```python
from build123d import *

# Parameters (mm, degrees)
SKETCH_1_W          = 220
SKETCH_1_H          = 45
EXTRUDE_1_DEPTH     = 6
EXTRUDE_2_DEPTH     = 35
SKETCH_5_W          = 4
SKETCH_5_H          = 3
CUT_EXTRUDE_3_DEPTH = 194.244663574
SKETCH_6_W          = 220
SKETCH_6_H          = 45
EXTRUDE_3_DEPTH     = 5
EXTRUDE_4_DEPTH     = 11
SKETCH_10_R         = 4.5
CUT_EXTRUDE_4_DEPTH = 172.992005628
FILLET_1_R          = 10
SKETCH_11_W         = 10
SKETCH_11_H         = 8
CUT_EXTRUDE_6_DEPTH = 35
SKETCH_18_W         = 228
SKETCH_18_H         = 45
EXTRUDE_5_DEPTH     = 1


with BuildPart() as part:
    # 草图1 → 凸台-拉伸1 (new body)
    with BuildSketch(Plane.XY):
        Rectangle(SKETCH_1_W, SKETCH_1_H)
    extrude(amount=EXTRUDE_1_DEPTH)

    # 草图2 → 凸台-拉伸2 (add)
    with BuildSketch(Plane.XY.offset(6)):
        Polygon((-77.5, 22.5), (77.5, 22.5), (77.5, 14.5), (75, 14.5), (-75, 14.5), (-77.5, 14.5), align=None)
        Polygon((-75, -14.5), (75, -14.5), (77.5, -14.5), (77.5, -22.5), (-77.5, -22.5), (-77.5, -14.5), align=None)
    extrude(amount=EXTRUDE_2_DEPTH)

    # 草图5 → 切除-拉伸3 (cut, through all)
    with BuildSketch(Plane.ZY.offset(77.5)):
        with Locations((11.5, -16)):
            Rectangle(SKETCH_5_W, SKETCH_5_H)
        with Locations((11.5, 16)):
            Rectangle(SKETCH_5_W, SKETCH_5_H)
    extrude(amount=-CUT_EXTRUDE_3_DEPTH, mode=Mode.SUBTRACT)

    # 草图6 → 凸台-拉伸3 (add)
    with BuildSketch(Plane(origin=(0, 0, 0), x_dir=(-1, 0, 0), z_dir=(0, 0, -1))):
        Rectangle(SKETCH_6_W, SKETCH_6_H)
    extrude(amount=EXTRUDE_3_DEPTH)

    # 草图9 → 凸台-拉伸4 (add)
    with BuildSketch(Plane(origin=(0, 0, -5), x_dir=(-1, 0, 0), z_dir=(0, 0, -1))):
        with BuildLine():
            Line((-110, -22.5), (-110, 22.5))
            Line((-110, 22.5), (-130, 22.5))
            Line((-130, 22.5), (-158.235294118, -30.441176471))
            ThreePointArc((-158.235294118, -30.441176471), (-152.058823529, -50.735294118), (-131.764705882, -44.558823529))
            Line((-131.764705882, -44.558823529), (-120, -22.5))
            Line((-120, -22.5), (-110, -22.5))
        make_face()
    extrude_4 = extrude(amount=-EXTRUDE_4_DEPTH)

    # 草图10 → 切除-拉伸4 (cut, through all)
    with BuildSketch(Plane.XY.offset(6)):
        with Locations((145, -37.5)):
            Circle(SKETCH_10_R)
    cut_extrude_4 = extrude(amount=-CUT_EXTRUDE_4_DEPTH, mode=Mode.SUBTRACT)

    # 镜向1: 凸台-拉伸4, 切除-拉伸4 across plane
    add(extrude_4.mirror(Plane(origin=(0, 0, 0), x_dir=(0, 0, 1), z_dir=(1, 0, 0))))
    add(cut_extrude_4.mirror(Plane(origin=(0, 0, 0), x_dir=(0, 0, 1), z_dir=(1, 0, 0))), mode=Mode.SUBTRACT)

    # 圆角1
    fillet_1_edges = [part.edges().sort_by_distance(p)[0] for p in [
        (-130, 22.5, 0.5),
        (-120, -22.5, 0.5),
        (130, 22.5, 0.5),
        (120, -22.5, 0.5),
    ]]
    fillet(fillet_1_edges, radius=FILLET_1_R)

    # 草图11 → 切除-拉伸6 (cut)
    with BuildSketch(Plane.XY.offset(41)):
        with Locations((-72.5, 18.5)):
            Rectangle(SKETCH_11_W, SKETCH_11_H)
        with Locations((72.5, 18.5)):
            Rectangle(SKETCH_11_W, SKETCH_11_H)
        with Locations((72.5, -18.5)):
            Rectangle(SKETCH_11_W, SKETCH_11_H)
        with Locations((-72.5, -18.5)):
            Rectangle(SKETCH_11_W, SKETCH_11_H)
    extrude(amount=-CUT_EXTRUDE_6_DEPTH, mode=Mode.SUBTRACT)

    # 草图18 → 凸台-拉伸5 (add)
    with BuildSketch(Plane(origin=(0, 0, -5), x_dir=(-1, 0, 0), z_dir=(0, 0, -1))):
        Rectangle(SKETCH_18_W, SKETCH_18_H)
    extrude(amount=EXTRUDE_5_DEPTH)


solid = part.part
```
Model file for the job. Use its own axes, mm. A direction names the side the tool comes from. Round coordinates to 2 decimals unless told otherwise and drop trailing zeros. Write each loop counter-clockwise with the first axis right and the second up, starting at its lowest first coordinate (ties: lowest second). Pieces come first, ordered by that corner, then holes. Notation, with made-up numbers: M 57,74 L 110,74 A13 cw 110,94 Z; hole C 56.25,69.25 d6. An arc over 180 degrees is marked long. Put each result on its own line as item: value.
Item 1: Tool access for faces 4 (the cylindrical face through (-119.21, -23.964, 0.577)), 5 (the flat face through (1, -14.5, 27)), 6 (the flat face through (67.5, -19, 24)): list every direction of +Z, -Z, +X, -X, +Y, -Y with a clear straight run to the whole face (end or side of a thin tool).
Responses:
face 4: +Z, -Z, -Y
face 5: +Z, +X, -X
face 6: +Z, +X, +Y, -Y
Item 2: Cut at D-D (x = 145). List the corners of the cut face in (y, z) (3 decimals), and give its area (3 significant figures).
Responses:
outline: M -52.5,-5 L -42,-5 L -42,6 L -52.5,6 Z; M -33,-5 L -5.625,-5 L -5.625,6 L -33,6 Z
area: 417 mm²
Item 3: Cut at C-C (z = 3). List the corners of the cut face in (x, y), and give its area (3 significant figures).
Responses:
outline: M -158.24,-30.44 A15 ccw -131.76,-44.56 L -122.82,-27.79 A10 cw -114,-22.5 L 114,-22.5 A10 cw 122.82,-27.79 L 131.76,-44.56 A15 ccw 158.24,-30.44 L 132.82,17.21 A10 ccw 124,22.5 L -124,22.5 A10 ccw -132.82,17.21 Z; hole C -145,-37.5 d9; hole C 145,-37.5 d9
area: 14,400 mm²
Item 4: Cut at B-B (y = -37.5). List the corners of the cut face in (x, z).
Responses:
outline: M -160,-5 L -149.5,-5 L -149.5,6 L -160,6 Z; M -140.5,-5 L -128,-5 L -128,6 L -140.5,6 Z; M 128,-5 L 140.5,-5 L 140.5,6 L 128,6 Z; M 149.5,-5 L 160,-5 L 160,6 L 149.5,6 Z
Item 5: Cut at A-A (z = 37). List the corners of the cut face in (x, y), and give its area (3 significant figures).
Responses:
outline: M -67.5,-22.5 L 67.5,-22.5 L 67.5,-14.5 L -67.5,-14.5 Z; M -67.5,14.5 L 67.5,14.5 L 67.5,22.5 L -67.5,22.5 Z
area: 2,160 mm²
Item 6: Flat gauge pins, fed straight in: P1, Ø14.5, axis at x = 145, y = -37.5, coming from the +Z side; P2, Ø4, axis at x = -51.5, z = 19, coming from the -Y side; P3, Ø2.5, axis at y = 19, z = 31, coming from the -X side. Where does each tip first touch, or does it go through?
Responses:
P1: z = 6
P2: y = -22.5
P3: x = -67.5
Item 7: Probe L1, parallel to Y at x = -2.5, z = 18.5; L2, parallel to X at y = -37, z = 2; L3, parallel to Z at x = -35.5, y = -15.5. List the from-to ranges inside material, lowest first. Write a range as from..to.
Responses:
L1: -22.5..-14.5, 14.5..22.5
L2: -159.99..-149.47, -140.53..-127.73, 127.73..140.53, 149.47..159.99
L3: -6..9.5, 13.5..41
Item 8: Mould opens along Y. For faces 1 (the flat face through (127.357, -36.294, 0.423)), 2 (the flat face through (-132, -14, -5)), 3 (the flat face through (-2, -6, 6)) say: +Y half, -Y half, draft (parallel to the pull), parting line (faces both ways), or undercut.
Responses:
face 1: -Y half
face 2: draft
face 3: undercut
